Build history of the part. All positions in model axes, mm. Face numbers are marked on the shaded views. Round coordinates to 2 decimals unless told otherwise and drop trailing zeros. Loops run counter-clockwise (first coordinate to the right, second up) from the corner with the lowest first, then second, coordinate; pieces in that order, holes last. Notation, with made-up numbers: M 66.25,69.25 L 97.25,69.25 A16 ccw 97.25,99.25 Z; hole C 14,-19 d4. An arc over 180 degrees is marked long. One line per item, written item: value.
Autodesk Inventor part; units mm, degrees
ref_plane "YZ Plane" through (0, 0, 0) normal (1, 0, 0) x (0, 1, 0)
ref_plane "XZ Plane" through (0, 0, 0) normal (0, 1, 0) x (-1, 0, 0)
ref_plane "XY Plane" through (0, 0, 0) normal (0, 0, 1) x (1, 0, 0)
sketch "Sketch1" plane through (0, 0, 0) normal (0, 0, 1) x (1, 0, 0)
  circle A0 centre (0, 0) radius 2
  circle A1 centre (0, 0) radius 1
  line L0 (0, 0) -> (22, 0)
  circle A2 centre (22, 0) radius 1
  circle A3 centre (22, 0) radius 2
  line L1 (0, 2) -> (22, 2)
  line L2 (0, -2) -> (22, -2)
  dimension "d0" = 4
  dimension "d1" = 2
  dimension "d2" = 22
  dimension "d3" = 2
  dimension "d4" = 4
extrude "Extrusion1" add sketch "Sketch1" along normal mid plane 2.6
sketch "Sketch3" plane through (0, 0, 0) normal (0, 0, 1) x (1, 0, 0)
  line L0 (0, 0) -> (4, 0)
  line L1 (4, 0) -> (4, 2)
  line L2 (22, 2) -> (0, 2)
  line L3 (4, 0) -> (4, -2)
  line L4 (0, -2) -> (22, -2)
  line L5 (4, 0) -> (20, 0)
  line L6 (20, 0) -> (20, 2)
  line L7 (20, 0) -> (20, -2)
  circle A0 centre (22, 0) radius 2.5
  point P0 (20, 1.5)
  point P1 (20, -1.5)
  dimension "d16" = 4
  dimension "d17" = 5
extrude "Extrusion3" add sketch "Sketch3" along normal mid plane 4.2 contours L5 A0 L7 L4 L3 | L1 L2 L6 A0 L5
fillet "Fillet3" radius 0.2 4 edges at (12, 2, 2.1) (12, -2, 2.1) (12, -2, -2.1) (12, 2, -2.1)
fillet "Fillet4" radius 0.1 20 edges at (20, 1.9414, 2.0414) (20, 2, 1.6) (20, 1.65, 2.1) (20, -1.65, 2.1) (20, -2, 1.6) (20, -1.9414, 2.0414) (20, 1.65, -2.1) (20, 2, -1.6) (20, 1.9414, -2.0414) (20, -1.9414, -2.0414) (20, -2, -1.6) (20, -1.65, -2.1) (4, 2, -1.6) (4, 0, -2.1) (4, -2, 1.6) (4, -2, -1.6) (4, 1.9414, -2.0414) (4, 1.9414, 2.0414) (4, 0, 2.1) (4, 2, 1.6)
properties part number "New_ThinArm_first"
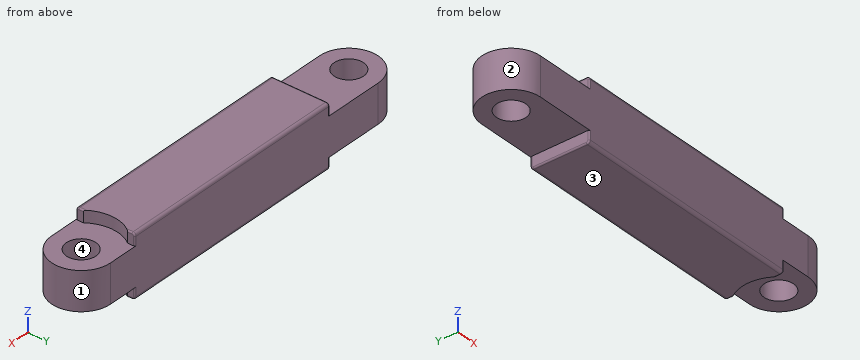
Item 1: Slice it at B-B, the plane z = 0.1. Give the cut face in (x, y).
Check values:
outline: M 0,-2 L 22,-2 A2 ccw 22,2 L 0,2 A2 ccw Z; hole C 0,0 d2; hole C 22,0 d2
Item 2: Slice it at C-C, the plane x = 2. Give the cut face in (y, z).
Check values:
outline: M -2,-1.3 L 2,-1.3 L 2,1.3 L -2,1.3 Z
Item 3: Drop flat-ended pins along their axis: P1, Ø1.2, axis at x = 0, y = 0, coming from the +Z side; P2, Ø2, axis at y = 1.5, z = 1.5, coming from the -X side; P3, Ø2, axis at x = 22.5, y = 0, coming from the +Z side; P4, Ø0.8, axis at y = 0.5, z = 1.5, coming from the -X side. Give the stop position or say it passes through.
Check values:
P1: passes through
P2: stops at x = -1.93
P3: stops at z = 1.3
P4: stops at x = -1.99
Item 4: Wall check: line 1 along X through (y, z) = (0.05, -0.8); line 2 along Y through (x, z) = (22, 0.5); line 3 along Z through (x, y) = (3.5, -1.65). Give the ranges that are in metal, low to high.
Check values:
line 1: x = -2 to -1, 1 to 21, 23 to 24
line 2: y = -2 to -1, 1 to 2
line 3: z = -1.3 to 1.3
Item 5: Slice it at A-A, the plane y = 0. Give the cut face in (x, z), and give its area (3 significant figures).
Check values:
outline: M -2,-1.3 L -1,-1.3 L -1,1.3 L -2,1.3 Z; M 1,-1.3 L 4,-1.3 L 4,-2 A0.1 ccw 4.1,-2.1 L 19.5,-2.1 L 19.5,-1.3 L 21,-1.3 L 21,1.3 L 19.5,1.3 L 19.5,2.1 L 4.1,2.1 A0.1 ccw 4,2 L 4,1.3 L 1,1.3 Z; M 23,-1.3 L 24,-1.3 L 24,1.3 L 23,1.3 Z
area: 82.0 mm2
Item 6: Pull direction X, two halves, no side cores. Call the marked faces 1, 2, 3 and 4: pulls with the +X half, pulls with the -X half, needs draft (parallel to the pull), parting line crosses it, or undercut.
Check values:
face 1: pulls with the +X half
face 2: pulls with the -X half
face 3: needs draft
face 4: undercut
